Autodesk Inventor part; units mm, degrees
ref_plane "bolt_XY" through (15, 0, 0) normal (1, 0, 0) x (0, 0, -1)
ref_plane "bolt_YZ" through (15, 0, 0) normal (0, 0, -1) x (0, 1, 0)
ref_plane "bolt_ZX" through (15, 0, 0) normal (0, 1, 0) x (1, 0, 0)
sketch "Sketch_1" plane through (0, 0, 0) normal (0, 0, 1) x (1, 0, 0)
  line L0 (15, 0) -> (-5, 0)
  line L1 (-5, 0) -> (-5, 3.75)
  line L2 (-5, 3.75) -> (-4.5, 4.25)
  line L3 (-4.5, 4.25) -> (0, 4.25)
  line L4 (0, 4.25) -> (0, 2.5)
  line L5 (0, 2.5) -> (14.5095, 2.5)
  line L6 (14.5095, 2.5) -> (15, 2.0095)
  line L7 (15, 2.0095) -> (15, 0)
  line L8 (15, 0) -> (-5, 0)
revolve "Revolution1" add sketch "Sketch_1" angle 360 about axis through (15, 0, 0) along (1, 0, 0)
thread "Thread1"
sketch "Sketch2" plane through (-5, 0, 0) normal (-1, 0, 0) x (0, 0, 1)
  point P0 (0, 0)
hole "Hole1" at (-5, 0, 0) direction (1, 0, 0) diameter 4 depth 2.5 tip angle 120
sketch "Sketch_3" plane through (-5, 0, 0) normal (1, 0, 0) x (0, 0, -1)
  line L0 (-2, -1.1547) -> (0, -2.3094)
  line L1 (0, -2.3094) -> (2, -1.1547)
  line L2 (2, -1.1547) -> (2, 1.1547)
  line L3 (2, 1.1547) -> (0, 2.3094)
  line L4 (0, 2.3094) -> (-2, 1.1547)
  line L5 (-2, 1.1547) -> (-2, -1.1547)
extrude "Extrusion1" cut sketch "Sketch_3" along normal blind 2.5
ref_plane "bolt_XY" through (15, 0, 0) normal (1, 0, 0) x (0, 0, -1)
ref_plane "bolt_YZ" through (15, 0, 0) normal (0, 0, -1) x (0, 1, 0)
ref_plane "bolt_ZX" through (15, 0, 0) normal (0, 1, 0) x (1, 0, 0)
ref_plane "nut_XY" through (0, 0, 0) normal (1, 0, 0) x (0, 0, -1)
ref_plane "nut_YZ" through (0, 0, 0) normal (0, 0, -1) x (0, 1, 0)
ref_plane "nut_ZX" through (0, 0, 0) normal (0, 1, 0) x (1, 0, 0)
properties part number "CBE5-15"
Work out the finished part from the listing and answer in its coordinate system (mm). A direction names the side the tool comes from. Give positions to 0.01 mm unless a question says otherwise; leave off trailing zeros. Write each loop counter-clockwise with the first axis right and the second up, starting at its lowest first coordinate (ties: lowest second). Pieces come first, ordered by that corner, then holes. Notation, with made-up numbers: (-9, 29.25) - (24, 29.25) arc R17 ccw to (24, 40.25) - close; hole circle Ø5 at (83, 64.25). An arc over 180 degrees is marked (long way). One line per item, written item: value. Start each with the question number.
1. Consider probe 1 along Z at (x, y) = (10.5, -1.5); probe 2 along Z at (x, y) = (5.5, 0); probe 3 along X at (y, z) = (2.5, -0.5). Determine where each line is inside the solid, lowest interval first.
2. Given pin 1 (1.1 mm diameter, centred on y = 0.5, z = 1.5, fed in from -X); pin 2 (4 mm diameter, centred on x = 7.5, y = 0.5, fed in from +Z); pin 3 (1 mm diameter, centred on x = 1, z = -2.5, fed in from +Y); pin 4 (0.7 mm diameter, centred on x = -4, y = -0.5, fed in from -Z), each flat-ended and moving along its own axis, determine where each tip first touches the part or whether it passes through.
3. Find section A-A (x = -0.75). Write down the section's boundary in (y, z), then the cut area to 3 significant figures.
4. For a pull along Z with two mould halves and no side action, classify faces 3 (the flat face through (-3.768, -1.724, 1.014)), 4 (the cylindrical face through (7.36, -0.54, -2.44)), 5 (the flat face through (0, 2, -2)) as +Z half, -Z half, draft (parallel to the pull), parting line (faces both ways), or undercut.
5. For faces 1 (the flat face through (-3.77, -1.74, -0.99)), 2 (the flat face through (15, 0, 0)), determine the directions among +Z, -Z, +X, -X, +Y, -Y from which every point of the face is accessible in a straight line to the end or side of a thin tool.
6. Find section B-B (x = 1.5). Write down the section's boundary in (y, z).
Geometry results:
1. probe 1: -2 to 2
1. probe 2: -2.5 to 2.5
1. probe 3: -5 to 0
2. pin 1: x = -5
2. pin 2: z = 2.5
2. pin 3: y = 1.5
2. pin 4: z = -4.25
3. outline: circle Ø8.5 at (0, 0)
3. area: 56.7 mm2
4. face 3: undercut
4. face 4: parting line
4. face 5: draft
5. face 1: -X
5. face 2: +Z, -Z, +X, +Y, -Y
6. outline: circle Ø5 at (0, 0)
